Geometry check sheet. Reference: the model listing, model coordinates, mm. Give positions to 0.01 mm unless a question says otherwise; leave off trailing zeros. Loops run counter-clockwise (first coordinate to the right, second up) from the corner with the lowest first, then second, coordinate; pieces in that order, holes last. Notation, with made-up numbers: (-9.75, 87) -> (8.25, 87) arc R26 cw to (8.25, 118) -> close; hole circle Ø8 at (44, -36.5). An arc over 180 degrees is marked (long way). One line per item, written item: value. Start each with the question number.
(1) Gauge pin test, flat end, axial feed: pin 1 Ø5 at (x, z) = (-7, -14.5) entering from +Y. Record the tip position at first contact, or that the pin passes through.
(2) Sectioned sample at B-B, the plane y = -2.2. State how many separate pieces and enclosed holes the cut face has, then the cut area to 3 significant figures.
(3) Scan lines: line 1 along X through (y, z) = (-1.1, -104); line 2 along Z through (x, y) = (-152.4, -1.1); line 3 along Z through (x, y) = (70, -0.5). Record each from-to range of solid material in increasing order. Write a range as from..to.
(4) Sectioned sample at A-A, the plane x = 12. Record the cut outline in (y, z) (3 decimals), then the cut area to 3 significant figures.
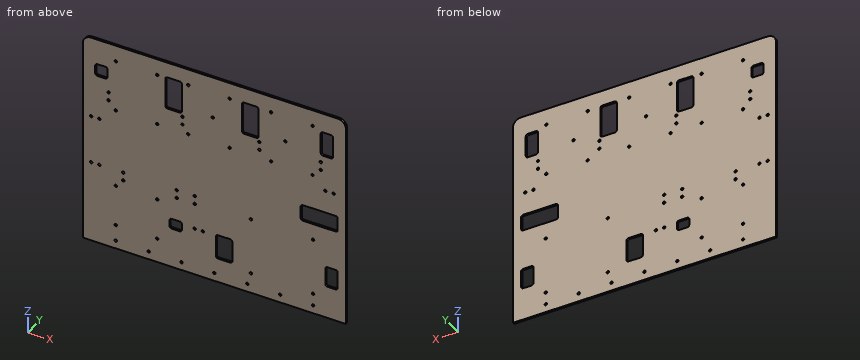
from build123d import *

# Parameters (mm, degrees)
F0_R     = 1.89865
F0_R_2   = 1.905
F1_DEPTH = 3.175


with BuildPart() as f1:
    # F0 (on Front) → F1 (new body)
    with BuildSketch(Plane.XZ):
        with BuildLine():
            Line((190.5, 165.1), (-190.5, 165.1))
            ThreePointArc((-190.5, 165.1), (-199.4802561211, 161.3802561211), (-203.2, 152.4))
            Line((-203.2, 152.4), (-203.2, -165.1))
            Line((-203.2, -165.1), (203.2, -165.1))
            Line((203.2, -165.1), (203.2, 152.4))
            ThreePointArc((203.2, 152.4), (199.4802561211, 161.3802561211), (190.5, 165.1))
        make_face()
        with Locations((-152.4, -152.4)):
            Circle(F0_R, mode=Mode.SUBTRACT)
        with Locations((-152.4, -127)):
            Circle(F0_R, mode=Mode.SUBTRACT)
        with Locations((-101.6, -152.4)):
            Circle(F0_R, mode=Mode.SUBTRACT)
        with Locations((-50.8, -152.4)):
            Circle(F0_R, mode=Mode.SUBTRACT)
        with Locations((-88.4, -127)):
            Circle(F0_R, mode=Mode.SUBTRACT)
        with Locations((0, -152.4)):
            Circle(F0_R, mode=Mode.SUBTRACT)
        with BuildLine():
            ThreePointArc((-69.35, -90.2375), (-68.4200640303, -87.9924359697), (-66.175, -87.0625))
            Line((-66.175, -87.0625), (-53.475, -87.0625))
            ThreePointArc((-53.475, -87.0625), (-51.2299359697, -87.9924359697), (-50.3, -90.2375))
            Line((-50.3, -90.2375), (-50.3, -99.7625))
            ThreePointArc((-50.3, -99.7625), (-51.2299359697, -102.0075640303), (-53.475, -102.9375))
            Line((-53.475, -102.9375), (-66.175, -102.9375))
            ThreePointArc((-66.175, -102.9375), (-68.4200640303, -102.0075640303), (-69.35, -99.7625))
            Line((-69.35, -99.7625), (-69.35, -90.2375))
        make_face(mode=Mode.SUBTRACT)
        with BuildLine():
            ThreePointArc((2.3, -92.075), (3.2299359697, -89.8299359697), (5.475, -88.9))
            Line((5.475, -88.9), (24.525, -88.9))
            ThreePointArc((24.525, -88.9), (26.7700640303, -89.8299359697), (27.7, -92.075))
            Line((27.7, -92.075), (27.7, -123.825))
            ThreePointArc((27.7, -123.825), (26.7700640303, -126.0700640303), (24.525, -127))
            Line((24.525, -127), (5.475, -127))
            ThreePointArc((5.475, -127), (3.2299359697, -126.0700640303), (2.3, -123.825))
            Line((2.3, -123.825), (2.3, -92.075))
        make_face(mode=Mode.SUBTRACT)
        with Locations((-30.4872877896, -90.7393252313)):
            Circle(F0_R_2, mode=Mode.SUBTRACT)
        with Locations((-17.7872877896, -90.7393252313)):
            Circle(F0_R_2, mode=Mode.SUBTRACT)
        with Locations((-152.4, -63)):
            Circle(F0_R, mode=Mode.SUBTRACT)
        with Locations((-190.5, -37.6)):
            Circle(F0_R_2, mode=Mode.SUBTRACT)
        with Locations((-177.8, -37.6)):
            Circle(F0_R_2, mode=Mode.SUBTRACT)
        with Locations((-140.8782303333, -50.3)):
            Circle(F0_R_2, mode=Mode.SUBTRACT)
        with Locations((-140.8782303333, -37.6)):
            Circle(F0_R_2, mode=Mode.SUBTRACT)
        with Locations((-88.4, -63)):
            Circle(F0_R, mode=Mode.SUBTRACT)
        with Locations((-58.2065284252, -50.3)):
            Circle(F0_R_2, mode=Mode.SUBTRACT)
        with Locations((-58.2065284252, -37.6)):
            Circle(F0_R_2, mode=Mode.SUBTRACT)
        with Locations((-30.4872877896, -50.3)):
            Circle(F0_R_2, mode=Mode.SUBTRACT)
        with Locations((-30.4872877896, -37.6)):
            Circle(F0_R_2, mode=Mode.SUBTRACT)
        with Locations((50.8, -152.4)):
            Circle(F0_R, mode=Mode.SUBTRACT)
        with Locations((56.4, -133.35)):
            Circle(F0_R, mode=Mode.SUBTRACT)
        with Locations((101.6, -152.4)):
            Circle(F0_R, mode=Mode.SUBTRACT)
        with Locations((152.4, -152.4)):
            Circle(F0_R, mode=Mode.SUBTRACT)
        with Locations((152.4, -133.35)):
            Circle(F0_R, mode=Mode.SUBTRACT)
        with BuildLine():
            ThreePointArc((171.45, -85.725), (172.3799359697, -83.4799359697), (174.625, -82.55))
            Line((174.625, -82.55), (187.325, -82.55))
            ThreePointArc((187.325, -82.55), (189.5700640303, -83.4799359697), (190.5, -85.725))
            Line((190.5, -85.725), (190.5, -111.125))
            ThreePointArc((190.5, -111.125), (189.5700640303, -113.3700640303), (187.325, -114.3))
            Line((187.325, -114.3), (174.625, -114.3))
            ThreePointArc((174.625, -114.3), (172.3799359697, -113.3700640303), (171.45, -111.125))
            Line((171.45, -111.125), (171.45, -85.725))
        make_face(mode=Mode.SUBTRACT)
        with Locations((56.4, -45.35)):
            Circle(F0_R, mode=Mode.SUBTRACT)
        with Locations((152.4, -45.35)):
            Circle(F0_R, mode=Mode.SUBTRACT)
        with BuildLine():
            ThreePointArc((133.35, 2.275), (134.2799359697, 4.5200640303), (136.525, 5.45))
            Line((136.525, 5.45), (187.325, 5.45))
            ThreePointArc((187.325, 5.45), (189.5700640303, 4.5200640303), (190.5, 2.275))
            Line((190.5, 2.275), (190.5, -16.775))
            ThreePointArc((190.5, -16.775), (189.5700640303, -19.0200640303), (187.325, -19.95))
            Line((187.325, -19.95), (136.525, -19.95))
            ThreePointArc((136.525, -19.95), (134.2799359697, -19.0200640303), (133.35, -16.775))
            Line((133.35, -16.775), (133.35, 2.275))
        make_face(mode=Mode.SUBTRACT)
        with Locations((-190.5, 37.1834747493)):
            Circle(F0_R_2, mode=Mode.SUBTRACT)
        with Locations((-177.8, 37.1834747493)):
            Circle(F0_R_2, mode=Mode.SUBTRACT)
        with Locations((-152.4, 59.7)):
            Circle(F0_R, mode=Mode.SUBTRACT)
        with Locations((-163.5061204433, 72.4)):
            Circle(F0_R_2, mode=Mode.SUBTRACT)
        with Locations((-163.5061204433, 85.1)):
            Circle(F0_R_2, mode=Mode.SUBTRACT)
        with Locations((-88.4, 59.7)):
            Circle(F0_R, mode=Mode.SUBTRACT)
        with Locations((-40.4, 59.7)):
            Circle(F0_R, mode=Mode.SUBTRACT)
        with Locations((-49.3557117879, 72.4)):
            Circle(F0_R_2, mode=Mode.SUBTRACT)
        with Locations((-49.3557117879, 85.1)):
            Circle(F0_R_2, mode=Mode.SUBTRACT)
        with BuildLine():
            ThreePointArc((-184.15, 122.05), (-183.2200640303, 124.2950640303), (-180.975, 125.225))
            Line((-180.975, 125.225), (-168.275, 125.225))
            ThreePointArc((-168.275, 125.225), (-166.0299359697, 124.2950640303), (-165.1, 122.05))
            Line((-165.1, 122.05), (-165.1, 109.35))
            ThreePointArc((-165.1, 109.35), (-166.0299359697, 107.1049359697), (-168.275, 106.175))
            Line((-168.275, 106.175), (-180.975, 106.175))
            ThreePointArc((-180.975, 106.175), (-183.2200640303, 107.1049359697), (-184.15, 109.35))
            Line((-184.15, 109.35), (-184.15, 122.05))
        make_face(mode=Mode.SUBTRACT)
        with Locations((-152.4, 139.7)):
            Circle(F0_R, mode=Mode.SUBTRACT)
        with BuildLine():
            ThreePointArc((-75.7, 137.925), (-74.7700640303, 140.1700640303), (-72.525, 141.1))
            Line((-72.525, 141.1), (-53.475, 141.1))
            ThreePointArc((-53.475, 141.1), (-51.2299359697, 140.1700640303), (-50.3, 137.925))
            Line((-50.3, 137.925), (-50.3, 93.475))
            ThreePointArc((-50.3, 93.475), (-51.2299359697, 91.2299359697), (-53.475, 90.3))
            Line((-53.475, 90.3), (-72.525, 90.3))
            ThreePointArc((-72.525, 90.3), (-74.7700640303, 91.2299359697), (-75.7, 93.475))
            Line((-75.7, 93.475), (-75.7, 137.925))
        make_face(mode=Mode.SUBTRACT)
        with Locations((-2.5362023386, 100.0438879837)):
            Circle(F0_R, mode=Mode.SUBTRACT)
        with Locations((-88.4, 139.7)):
            Circle(F0_R, mode=Mode.SUBTRACT)
        with Locations((-40.4, 139.7)):
            Circle(F0_R, mode=Mode.SUBTRACT)
        with Locations((23.6, 59.7)):
            Circle(F0_R, mode=Mode.SUBTRACT)
        with Locations((69.5100128651, 72.4)):
            Circle(F0_R_2, mode=Mode.SUBTRACT)
        with Locations((69.5100128651, 85.1)):
            Circle(F0_R_2, mode=Mode.SUBTRACT)
        with Locations((87.6, 59.7)):
            Circle(F0_R, mode=Mode.SUBTRACT)
        with Locations((171.45, 40.65)):
            Circle(F0_R_2, mode=Mode.SUBTRACT)
        with Locations((184.15, 40.65)):
            Circle(F0_R_2, mode=Mode.SUBTRACT)
        with Locations((151.6, 59.7)):
            Circle(F0_R, mode=Mode.SUBTRACT)
        with Locations((164.3778979778, 72.4)):
            Circle(F0_R_2, mode=Mode.SUBTRACT)
        with Locations((164.3778979778, 85.1)):
            Circle(F0_R_2, mode=Mode.SUBTRACT)
        with BuildLine():
            ThreePointArc((42.65, 137.925), (43.5799359697, 140.1700640303), (45.825, 141.1))
            Line((45.825, 141.1), (64.875, 141.1))
            ThreePointArc((64.875, 141.1), (67.1200640303, 140.1700640303), (68.05, 137.925))
            Line((68.05, 137.925), (68.05, 93.475))
            ThreePointArc((68.05, 93.475), (67.1200640303, 91.2299359697), (64.875, 90.3))
            Line((64.875, 90.3), (45.825, 90.3))
            ThreePointArc((45.825, 90.3), (43.5799359697, 91.2299359697), (42.65, 93.475))
            Line((42.65, 93.475), (42.65, 137.925))
        make_face(mode=Mode.SUBTRACT)
        with Locations((109.4637976614, 100.0438879837)):
            Circle(F0_R, mode=Mode.SUBTRACT)
        with Locations((23.6, 139.7)):
            Circle(F0_R, mode=Mode.SUBTRACT)
        with Locations((87.6, 139.7)):
            Circle(F0_R, mode=Mode.SUBTRACT)
        with BuildLine():
            ThreePointArc((164.3, 131.575), (165.2299359697, 133.8200640303), (167.475, 134.75))
            Line((167.475, 134.75), (180.175, 134.75))
            ThreePointArc((180.175, 134.75), (182.4200640303, 133.8200640303), (183.35, 131.575))
            Line((183.35, 131.575), (183.35, 99.825))
            ThreePointArc((183.35, 99.825), (182.4200640303, 97.5799359697), (180.175, 96.65))
            Line((180.175, 96.65), (167.475, 96.65))
            ThreePointArc((167.475, 96.65), (165.2299359697, 97.5799359697), (164.3, 99.825))
            Line((164.3, 99.825), (164.3, 131.575))
        make_face(mode=Mode.SUBTRACT)
        with Locations((151.6, 139.7)):
            Circle(F0_R, mode=Mode.SUBTRACT)
    extrude(amount=F1_DEPTH)


solid = f1.part
Calculated:
1. pin 1: stops at y = 0
2. separate pieces: 1
2. enclosed holes: 59
2. area: 127,000 mm2
3. line 1: x = -203.2..2.3, 27.7..171.45, 190.5..203.2
3. line 2: z = -165.1..-154.3, -150.5..-128.9, -125.1..-64.9, -61.1..57.8, 61.6..137.8, 141.6..165.1
3. line 3: z = -165.1..70.56, 74.24..83.26, 86.94..165.1
4. outline: (-3.175, -165.1) -> (0, -165.1) -> (0, -127) -> (-3.175, -127) -> close; (-3.175, -88.9) -> (0, -88.9) -> (0, 165.1) -> (-3.175, 165.1) -> close
4. area: 927 mm2
